Part model, mm, in its own coordinate system. A direction names the side the tool comes from. Coordinates: 2 decimals unless noted, no trailing zeros. Order: outer loops, then holes, each group sorted by start corner. A loop starts at its lowest first (then second) coordinate and runs counter-clockwise, first axis right, second up.
```python
from build123d import *

# Parameters (mm, degrees)
SKETCH2_W           = 45
SKETCH2_H           = 20
BOSS_EXTRUDE1_DEPTH = 8
SKETCH3_W           = 25
SKETCH3_H           = 20
BOSS_EXTRUDE2_DEPTH = 30
SKETCH4_R           = 2.5
CUT_EXTRUDE1_DEPTH  = 8
SKETCH5_R           = 9.5
CUT_EXTRUDE2_DEPTH  = 20
FILLET2_RADIUS      = 12.5
FILLET2_LENGTH      = 20


with BuildPart() as part:
    # Sketch2 → Boss-Extrude1 (new body)
    with BuildSketch(Plane(origin=(0, 0, 0), x_dir=(1, 0, 0), z_dir=(0, 1, 0))):
        Rectangle(SKETCH2_W, SKETCH2_H)
    extrude(amount=BOSS_EXTRUDE1_DEPTH)

    # Sketch3 → Boss-Extrude2 (add)
    with BuildSketch(Plane(origin=(0, 8, 0), x_dir=(1, 0, 0), z_dir=(0, 1, 0))):
        Rectangle(SKETCH3_W, SKETCH3_H)
    extrude(amount=BOSS_EXTRUDE2_DEPTH)

    # Sketch4 → Cut-Extrude1 (cut)
    with BuildSketch(Plane(origin=(0, 8, 0), x_dir=(1, 0, 0), z_dir=(0, 1, 0))):
        with Locations(Location((-17.5, 0, 0), (0, 0, 270))):
            Circle(SKETCH4_R)
        with Locations(Location((17.5, 0, 0), (0, 0, 270))):
            Circle(SKETCH4_R)
    extrude(amount=-CUT_EXTRUDE1_DEPTH, mode=Mode.SUBTRACT)

    # Sketch5 → Cut-Extrude2 (cut)
    with BuildSketch(Plane.XY.offset(10)):
        with Locations((0, 23)):
            Circle(SKETCH5_R)
    extrude(amount=-CUT_EXTRUDE2_DEPTH, mode=Mode.SUBTRACT)

    # Fillet2: full round fillet: the end face becomes a half cylinder, R = half its width
    fillet2_face = Plane((0, 38, 0), x_dir=(0, 0, -1), z_dir=(0, 1, 0))  # on the end face: x along it, z out of the body
    fillet2_slab = fillet2_face.offset(-FILLET2_RADIUS / 2) * Box(FILLET2_LENGTH, 2 * FILLET2_RADIUS, FILLET2_RADIUS, mode=Mode.PRIVATE)  # the body's end, R deep
    fillet2_round = Plane((0, 25.5, 0), x_dir=(0, 1, 0), z_dir=(0, 0, -1)) * Cylinder(FILLET2_RADIUS, FILLET2_LENGTH, mode=Mode.PRIVATE)  # its axis R under the face
    add(fillet2_slab - fillet2_round, mode=Mode.SUBTRACT)


solid = part.part
```
(1) Slice it at D-D, the plane z = 3. Give the cut face in (x, y).
(2) Slice it at B-B, the plane x = 19.5. Give the cut face in (y, z).
(3) Tool access for faces 1 (the face through (0, 38, 0)), 2 (the face through (12.5, 17, 0)), 3 (the face through (-18.7, 8, -2.4)): list every direction of +Z, -Z, +X, -X, +Y, -Y with a clear straight run to the whole face (end or side of a thin tool).
(4) Pull direction Z, two halves, no side cores. Call faces 4 (the face through (-22.5, 4, 0)), 5 (the face through (0, 10, -10)), 6 (the face through (20, 4, 0)), 7 (the face through (-19.94, 4.06, -0.54)): +Z half, -Z half, draft (parallel to the pull), parting line (faces both ways), or undercut.
(5) Slice it at A-A, the plane z = 0. Give the cut face in (x, y).
(6) Probe line 1 (X direction, y = 3.5, z = 0); line 2 (X direction, y = 7, z = -2.25); line 3 (Y direction, x = 0, z = -0.25). List the from-to ranges inside material, lowest first.
(7) Drop flat-ended pins along their axis: pin 1 (6 mm diameter, centred on x = 0.5, z = -6, fed in from +Y); pin 2 (10 mm diameter, centred on y = 23, z = -5, fed in from +X); pin 3 (3 mm diameter, centred on x = 17.5, z = 0, fed in from -Y); pin 4 (11 mm diameter, centred on x = 15, z = 3, fed in from +Y). Give the stop position or say it passes through.
(8) Slice it at C-C, the plane y = 23. Give the cut face in (x, z), then the cut area to 3 significant figures.
Here are the results:
1. outline: (-22.5, 0) - (22.5, 0) - (22.5, 8) - (12.5, 8) - (12.5, 25.5) arc R12.5 ccw to (-12.5, 25.5) - (-12.5, 8) - (-22.5, 8) - close; hole circle Ø19 at (0, 23)
2. outline: (0, -10) - (8, -10) - (8, -1.5) - (0, -1.5) - close; (0, 1.5) - (8, 1.5) - (8, 10) - (0, 10) - close
3. face 1: +Z, -Z, +Y
3. face 2: +Z, -Z, +X, +Y
3. face 3: +Z, -Z, -X, +Y
4. face 4: draft
4. face 5: -Z half
4. face 6: undercut
4. face 7: undercut
5. outline: (-22.5, 0) - (-20, 0) - (-20, 8) - (-22.5, 8) - close; (-15, 0) - (15, 0) - (15, 8) - (12.5, 8) - (12.5, 25.5) arc R12.5 ccw to (-12.5, 25.5) - (-12.5, 8) - (-15, 8) - close; (20, 0) - (22.5, 0) - (22.5, 8) - (20, 8) - close; hole circle Ø19 at (0, 23)
6. line 1: x = -22.5 to -20, -15 to 15, 20 to 22.5
6. line 2: x = -22.5 to -18.59, -16.41 to 16.41, 18.59 to 22.5
6. line 3: y = 0 to 13.5, 32.5 to 38
7. pin 1: stops at y = 38
7. pin 2: stops at x = 12.5
7. pin 3: passes through
7. pin 4: stops at y = 33.62
8. outline: (-12.5, -10) - (-9.5, -10) - (-9.5, 10) - (-12.5, 10) - close; (9.5, -10) - (12.5, -10) - (12.5, 10) - (9.5, 10) - close
8. area: 120 mm2
